Input: part model. Units: mm. Frame: model coordinates. A direction names the side the tool comes from. Coordinates: 2 decimals unless noted, no trailing zeros. Order: outer loops, then holes, each group sorted by start corner. A loop starts at its lowest first (then second) coordinate and runs counter-clockwise, first axis right, second up. Notation, with made-up numbers: (11.25, -13.5) -> (46.25, -13.5) arc R24 cw to (46.25, 2.5) -> close; hole circle Ø1 at (-33.75, -1.75). An arc over 180 degrees is marked (long way). Write each question's results on one line, items separated by ' | '.
Autodesk Inventor part; units mm, degrees
ref_plane "YZ Plane" through (0, 0, 0) normal (1, 0, 0) x (0, 1, 0)
ref_plane "XZ Plane" through (0, 0, 0) normal (0, 1, 0) x (-1, 0, 0)
ref_plane "XY Plane" through (0, 0, 0) normal (0, 0, 1) x (1, 0, 0)
sketch "Boceto1" plane through (0, 0, 0) normal (0, 1, 0) x (-1, 0, 0)
  line L0 (9.9, 20.3) -> (-9.9, 20.3)
  line L1 (-9.9, 20.3) -> (-9.9, -20.3)
  line L2 (-9.9, -20.3) -> (9.9, -20.3)
  line L3 (9.9, -20.3) -> (9.9, 20.3)
  line L4 (9.9, 20.3) -> (-9.9, -20.3) construction
  line L5 (-9.9, 20.3) -> (9.9, -20.3) construction
  point P0 (0, 0)
  dimension "d0" = 19.8
  dimension "d1" = 40.6
extrude "Extrusión1" add sketch "Boceto1" against normal blind 9
sketch "Boceto2" plane through (0, 0, 0) normal (0, 1, 0) x (1, 0, 0)
  circle A0 centre (0, 10.3) radius 3
  line L0 (9.9, 20.3) -> (-9.9, 20.3)
  point P0 (0, 0)
  dimension "d4" = 6
  dimension "d5" = 10
extrude "Extrusión2" cut sketch "Boceto2" against normal through all
sketch "Boceto5" plane through (0, -9, 0) normal (0, -1, 0) x (1, 0, 0)
  line L0 (-8.9, 20.3) -> (8.9, 20.3)
  line L1 (8.9, 20.3) -> (8.9, 27.3)
  line L2 (8.9, 27.3) -> (-8.9, 27.3)
  line L3 (-8.9, 27.3) -> (-8.9, 20.3)
  line L4 (-8.9, 20.3) -> (8.9, 27.3) construction
  line L5 (8.9, 20.3) -> (-8.9, 27.3) construction
  line L6 (-9.9, 27.3) -> (9.9, 27.3)
  line L7 (9.9, 20.3) -> (-9.9, 20.3)
  point P0 (0, 0)
  point P1 (0, 0)
  point P2 (0, 23.8)
  dimension "d23" = 17.8
  dimension "d24" = 7
extrude "Extrusión5" add sketch "Boceto5" against normal blind 2.8
sketch "Boceto6" plane through (0, -6.2, 0) normal (0, 1, 0) x (1, 0, 0)
  arc A0 (-3.75, -26.7004) -> (-6.25, -26.7004) centre (-5, -24.89) ccw
  line L0 (-8.9, -27.3) -> (8.9, -27.3)
  line L1 (-3.75, -27.3) -> (-6.25, -27.3)
  line L2 (-6.25, -27.3) -> (-6.25, -26.7)
  line L3 (-3.75, -26.7) -> (-3.75, -27.3)
  line L4 (0, -27.3) -> (0, -23.9124)
  line L5 (-8.9, -20.3) -> (-8.9, -27.3)
  line L6 (-8.9, -20.3) -> (8.9, -20.3)
  line L7 (-8.3229, -20.3) -> (8.9, -20.3)
  line L8 (8.9, -20.3) -> (8.9, -27.3)
  point P0 (0, 0)
  point P1 (0, 0)
  dimension "d27" = 4.4
  dimension "d28" = 2.41
  dimension "d29" = 5
  dimension "d30" = 2.65
  dimension "d31" = 0.6
extrude "Extrusión6" cut sketch "Boceto6" against normal through all contours L3 L0 L2 A0
sketch "Boceto8" plane through (0, 0, 0) normal (1, 0, 0) x (0, 1, 0)
  line L0 (-6.2, 27.3) -> (-5.4, 20.3)
  line L1 (-5.4, 20.3) -> (-6.2, 20.3)
  line L2 (-6.2, 20.3) -> (-6.2, 27.3)
  point P0 (0, 0)
  dimension "d34" = 0.8
extrude "Extrusión7" add sketch "Boceto8" along normal mid plane 1
mirror "Simetría3" about plane through (0, 0, 0) normal (1, 0, 0) of "Extrusión6"
mirror "Simetría4" about plane through (0, 0, 0) normal (0, 0, 1) of "Extrusión5", "Extrusión6", "Simetría3", "Extrusión7"
sketch "Boceto9" plane through (0, 0, 0) normal (0, 1, 0) x (1, 0, 0)
  circle A0 centre (0, 10.3) radius 3
  line L0 (-8.9, -13.5986) -> (8.9, -13.5986)
  line L1 (8.9, -13.5986) -> (8.9, 6.7014)
  line L2 (-8.9, 6.7014) -> (-8.9, -13.5986)
  line L3 (-8.9, -13.5986) -> (5.885, 8.9919) construction
  line L4 (8.9, -13.5986) -> (-5.885, 8.9919) construction
  arc A1 (8.9, 6.7014) -> (-8.9, 6.7014) centre (0, 10.3) ccw
  line L5 (9.9, 20.3) -> (-9.9, 20.3)
  point P0 (0, 0)
  dimension "d40" = 9.6
  dimension "d42" = 20.3
  dimension "d61" = 17.8
extrude "Extrusión8" add sketch "Boceto9" along normal blind 2
sketch "Boceto11" plane through (0, 2, 0) normal (0, 1, 0) x (1, 0, 0)
  line L0 (-8.9, -13.5986) -> (8.9, -13.5986)
  line L1 (5.2244, -15.7986) -> (5.2244, -13.5986)
  arc A0 (-4.1756, -13.5986) -> (5.2244, -13.5986) centre (0.5244, -9.6782) ccw
  line L2 (-4.1756, -13.5986) -> (5.2244, -13.5986)
  point P0 (0, 0)
  dimension "d50" = 2.2
  dimension "d51" = 9.4
extrude "Extrusión9" add sketch "Boceto11" against normal blind 2
sketch "Boceto12" plane through (0, 2, 0) normal (0, 1, 0) x (1, 0, 0)
  circle A0 centre (0, 10.3) radius 6.4
  circle A1 centre (0, 10.3) radius 3
  point P0 (0, 0)
  dimension "d54" = 12.8
extrude "Extrusión10" add sketch "Boceto12" along normal blind 1.3
sketch "Boceto13" plane through (0, 3.3, -10.3) normal (0, 1, 0) x (1, 0, 0)
  circle A0 centre (0, 0) radius 5.6
  circle A1 centre (0, 0) radius 3
  point P0 (0, -10.3)
  dimension "d57" = 11.2
extrude "Extrusión11" add sketch "Boceto13" along normal blind 0.9
sketch "Boceto15" plane through (0, 2, 0) normal (0, 1, 0) x (1, 0, 0)
  line L0 (8.9, 6.7014) -> (8.9, -13.5986)
  line L1 (-8.9, -13.5986) -> (8.9, -13.5986)
  line L2 (8.9, -13.5986) -> (8.9, -1.0986)
  line L3 (8.9, -1.0986) -> (-8.9, -1.0986)
  line L4 (-8.9, -1.0986) -> (-8.9, -13.5986)
  line L5 (-8.9, -13.5986) -> (8.9, -1.0986) construction
  line L6 (8.9, -13.5986) -> (-8.9, -1.0986) construction
  line L7 (-8.9, -13.5986) -> (-4.1756, -13.5986)
  line L8 (-7.8, -12.4986) -> (7.8, -12.4986)
  line L9 (7.8, -12.4986) -> (7.8, -2.1986)
  line L10 (7.8, -2.1986) -> (-7.8, -2.1986)
  line L11 (-7.8, -2.1986) -> (-7.8, -12.4986)
  point P0 (0, 0)
  point P1 (0, -7.3486)
  dimension "d62" = 12.5
  dimension "d63" = 1.1
extrude "Extrusión12" add sketch "Boceto15" along normal blind 0.3
sketch "Boceto16" plane through (0, 2.3, 0) normal (0, 1, 0) x (1, 0, 0)
  arc A0 (1.91, -1.0986) -> (-1.91, -1.0986) centre (0, -0.7586) ccw
  line L0 (-7.8, -2.1986) -> (7.8, -2.1986)
  line L1 (8.9, -1.0986) -> (-8.9, -1.0986)
  point P0 (0, 0)
  dimension "d66" = 3.88
  dimension "d67" = 1.44
extrude "Extrusión13" add sketch "Boceto16" against normal blind 0.3
sketch "Boceto17" plane through (0, 0, 0) normal (0, 1, 0) x (1, 0, 0)
  line L0 (-9.9, 20.3) -> (-9.9, -20.3)
  line L1 (9.9, -20.3) -> (9.9, 20.3)
  line L2 (-9.9, -20.3) -> (9.9, -20.3)
  line L3 (9.9, 20.3) -> (-9.9, 20.3)
  line L4 (-9.6, -20) -> (-9.6, 20)
  line L5 (-9.6, 20) -> (9.6, 20)
  line L6 (9.6, 20) -> (9.6, -20)
  line L7 (9.6, -20) -> (-9.6, -20)
  point P0 (0, 0)
  dimension "d70" = 0.3
extrude "Extrusión14" cut sketch "Boceto17" against normal blind 0.5
fillet "Empalme1" radius 1 10 edges at (9.9, -4.75, 20.3) (8.9, -7.6, 27.3) (-8.9, -7.6, 27.3) (-9.9, -4.75, 20.3) (8.9, 1.15, 13.5986) (-8.9, 1.15, 13.5986) (9.9, -4.75, -20.3) (-9.9, -4.75, -20.3) (-8.9, -7.6, -27.3) (8.9, -7.6, -27.3)
fillet "Empalme2" radius 0.7 4 edges at (9.6, -0.25, 20) (-9.6, -0.25, 20) (9.6, -0.25, -20) (-9.6, -0.25, -20)
sketch "Boceto18" plane through (0, 2, 0) normal (0, 1, 0) x (1, 0, 0)
  point P0 (0, 0)
properties part number "Top" material "Plástico ABS"
(1) Cut plane A-A, the plane y = -4.5. Return loops of the section in (x, z), plus the area to 3 significant figures.
Return value:
outline: (-9.9, -19.3) arc R1 ccw to (-8.9, -20.3) -> (8.9, -20.3) arc R1 ccw to (9.9, -19.3) -> (9.9, 19.3) arc R1 ccw to (8.9, 20.3) -> (-8.9, 20.3) arc R1 ccw to (-9.9, 19.3) -> close; hole circle Ø6 at (0, -10.3) | area: 775 mm2
(2) Reachability of faces 1 (the face through (0, 2.3, 2)), 2 (the face through (2.9, 0, -19.8)), 3 (the face through (8.9, -8, 23)), 4 (the face through (0.45, 1.01, 15.8)), 5 (the face through (8.9, 1, 3)) from +Z, -Z, +X, -X, +Y, -Y: full face, straight path, thin tool, end or side. Return the list, or none.
Return value:
face 1: +Z, +X, -X, +Y | face 2: -Z, +Y | face 3: +Z, +X, +Y, -Y | face 4: +Z, +Y | face 5: +Z, +X, +Y
(3) Pin query (flat end, axial travel): P1, Ø6, axis at x = -7, y = -2, coming from the +Z side; P2, Ø0.5, axis at y = -7.5, z = 27, coming from the -X side; P3, Ø5.5, axis at x = 5, z = -24.89, coming from the +Y side. Return the tip coordinate at first contact, or that it passes through.
Return value:
P1: z = 20.3 | P2: x = -8.79 | P3: y = -6.2
(4) Line query: line 1 along X through (y, z) = (-8.25, -24.89); line 2 along X through (y, z) = (-7.75, -10.5); line 3 along Z through (x, y) = (8.5, -5.5). Output: solid intervals per line, ascending. Write a range as from..to.
Return value:
line 1: -8.9..-7.2, -2.8..2.8, 7.2..8.9 | line 2: -9.9..-2.99, 2.99..9.9 | line 3: -20.3..20.3
(5) Cut plane B-B, the plane z = -24.89. Return loops of the section in (x, y), plus the area to 3 significant figures.
Return value:
outline: (-8.9, -9) -> (-7.2, -9) -> (-7.2, -6.2) -> (-8.9, -6.2) -> close; (-2.8, -9) -> (2.8, -9) -> (2.8, -6.2) -> (0.5, -6.2) -> (0.5, -5.92) -> (-0.5, -5.92) -> (-0.5, -6.2) -> (-2.8, -6.2) -> close; (7.2, -9) -> (8.9, -9) -> (8.9, -6.2) -> (7.2, -6.2) -> close | area: 25.5 mm2
(6) Mould query, pull axis X, two halves, no side actions, for faces 6 (the face through (4.92, -7.58, -22.69)), 7 (the face through (-0.729, 3.744, -4.748)), 8 (the face through (-7, -8, -27.3)), 9 (the face through (0, 2, 7)). Classes: +X half, -X half, draft (parallel to the pull), parting line (faces both ways), or undercut.
Return value:
face 6: undercut | face 7: parting line | face 8: draft | face 9: undercut
